from build123d import *

# Parameters (mm, degrees)
SKETCH_2_R               = 4
CUT_EXTRUDE_1_DEPTH      = 152.843669608
PATTERN_CIRCULAR_1_COUNT = 4
SKETCH_4_W               = 12
SKETCH_4_H               = 23.3
CUT_EXTRUDE_2_DEPTH      = 202.961630019


with BuildPart() as part:
    # Эскиз1 → Повернуть1 (revolve)
    with BuildSketch(Plane.XY, mode=Mode.PRIVATE) as revolve_1_sk:
        Polygon((-5, 20), (-5, 30), (-41.5, 30), (-41.5, 40.016205048), (41.5, 40.016205048), (41.5, 30), (5, 30), (5, 20), (87, 20), (87, 30), (42.5, 30), (42.5, 50), (25, 50), (25, 72.5), (-25, 72.5), (-25, 50), (-42.5, 50), (-42.5, 30), (-87, 30), (-87, 20), align=None)
    revolve(revolve_1_sk.sketch.rotate(Axis((-171.104100946, 0, 0), (1, 0, 0)), 90), axis=Axis((-171.104100946, 0, 0), (1, 0, 0)))

    # Эскиз2 → Вырез-Вытянуть1 (cut, through all)
    with BuildSketch(Plane(origin=(25, 0, 0), x_dir=(0, 0, -1), z_dir=(1, 0, 0))):
        with Locations((0, 61.25)):
            Circle(SKETCH_2_R)
    cut_extrude_1 = extrude(amount=-CUT_EXTRUDE_1_DEPTH, mode=Mode.SUBTRACT)

    # Круговой массив1: Вырез-Вытянуть1 ×4 about axis
    pattern_circular_1_axis = Axis((0, 0, 0), (1, 0, 0))
    for i in range(1, PATTERN_CIRCULAR_1_COUNT):
        add(cut_extrude_1.rotate(pattern_circular_1_axis, i * 360 / PATTERN_CIRCULAR_1_COUNT), mode=Mode.SUBTRACT)

    # Эскиз4 → Вырез-Вытянуть2 (cut, through all)
    with BuildSketch(Plane.ZY.offset(87)):
        with Locations((0, -11.65)):
            Rectangle(SKETCH_4_W, SKETCH_4_H)
    extrude(amount=-CUT_EXTRUDE_2_DEPTH, mode=Mode.SUBTRACT)


solid = part.part
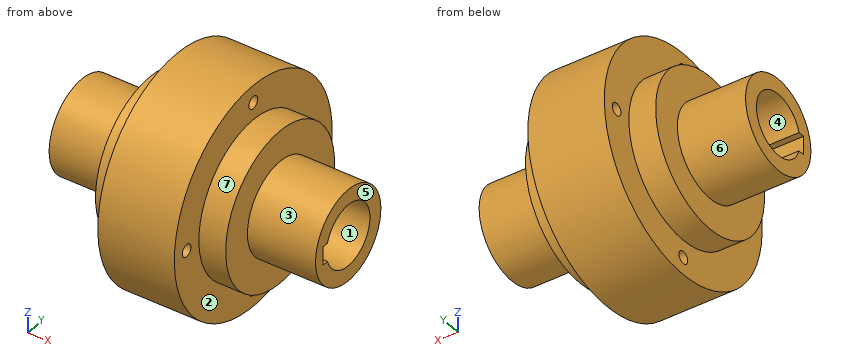
Source: CAD feature listing. Evaluate the final solid. Frame: model axes, mm. Face numbers are marked on the shaded views. A direction names the side the tool comes from. Coordinates: 2 decimals unless noted, no trailing zeros. Order: outer loops, then holes, each group sorted by start corner. A loop starts at its lowest first (then second) coordinate and runs counter-clockwise, first axis right, second up. Notation, with made-up numbers: M -25,11 L -21,11 A27 cw -21,31 Z; hole C 66.25,-37 d8. An arc over 180 degrees is marked long. Write each question's results on one line, items separated by ' | '. Start each with the question number.
1. Pin query (flat end, axial travel): pin 1 (4 mm diameter, centred on x = -60, y = 14, fed in from -Z); pin 2 (10.5 mm diameter, centred on y = 0, z = -61.25, fed in from +X); pin 3 (2 mm diameter, centred on x = 16, z = 46.5, fed in from +Y). Return the tip coordinate at first contact, or that it passes through.
2. Draft query along Y for the marked faces 1, 2, 3 and 4. Return one class per face: +Y half, -Y half, draft (parallel to the pull), parting line (faces both ways), or undercut.
3. Section B-B, the plane z = -61.25. Return the cut outline in (x, y).
4. Section A-A, the plane x = 14.5. Return the cut outline in (y, z), then the cut area to 3 significant figures.
5. Reachability of the marked faces 5, 6 and 7 from +Z, -Z, +X, -X, +Y, -Y: full face, straight path, thin tool, end or side. Return the list, or none.
6. Material intervals for L1, parallel to Y at x = 13, z = 0; L2, parallel to X at y = -4.5, z = 39; L3, parallel to Y at x = -10, z = -13, sorted ascending.
7. Section D-D, the plane z = -36.5. Return the cut outline in (x, y).
Solution:
1) pin 1: z = -27.5 | pin 2: x = 25 | pin 3: y = 56.44
2) face 1: undercut | face 2: draft | face 3: parting line | face 4: undercut
3) outline: M -25,-38.79 L 25,-38.79 L 25,-4 L -25,-4 Z; M -25,4 L 25,4 L 25,38.79 L -25,38.79 Z
4) outline: C 0,0 d145; C 0,0 d60; hole C -61.25,0 d8; hole C 0,0 d80.03; hole M -23.3,-6 L -19.08,-6 A20 ccw long -19.08,6 L -23.3,6 Z; hole C 0,-61.25 d8; hole C 0,61.25 d8; hole C 61.25,0 d8 | area: 12,800 mm²
5) face 5: +Z, -Z, +X, +Y, -Y | face 6: -X | face 7: +X
6) L1: -72.5 to -65.25, -57.25 to -40.02, -30 to -23.3, 20 to 30, 40.02 to 57.25, 65.25 to 72.5 | L2: -42.5 to -41.5, 41.5 to 42.5 | L3: -71.32 to -37.85, -27.04 to -15.2, 15.2 to 27.04, 37.85 to 71.32
7) outline: M -42.5,-34.17 L -25,-34.17 L -25,-62.64 L 25,-62.64 L 25,-34.17 L 42.5,-34.17 L 42.5,34.17 L 25,34.17 L 25,62.64 L -25,62.64 L -25,34.17 L -42.5,34.17 Z; hole M -41.5,-16.4 L 41.5,-16.4 L 41.5,16.4 L -41.5,16.4 Z
